Geometry check sheet. Reference: drawing and pictorial views, mm from the part's lowest x, y, z. A direction names the side the tool comes from. Coordinates: 2 decimals unless noted, no trailing zeros. Loops run counter-clockwise (first coordinate to the right, second up) from the corner with the lowest first, then second, coordinate; pieces in that order, holes last. Notation, with made-up numbers: (-10.75, 74) -> (-5.75, 74) arc R24 ccw to (-5.75, 106) -> close; hole circle Ø5 at (-22.5, 72). An arc over 180 degrees is marked (long way). Use CSV: the item, a comma, the result in double quotes.
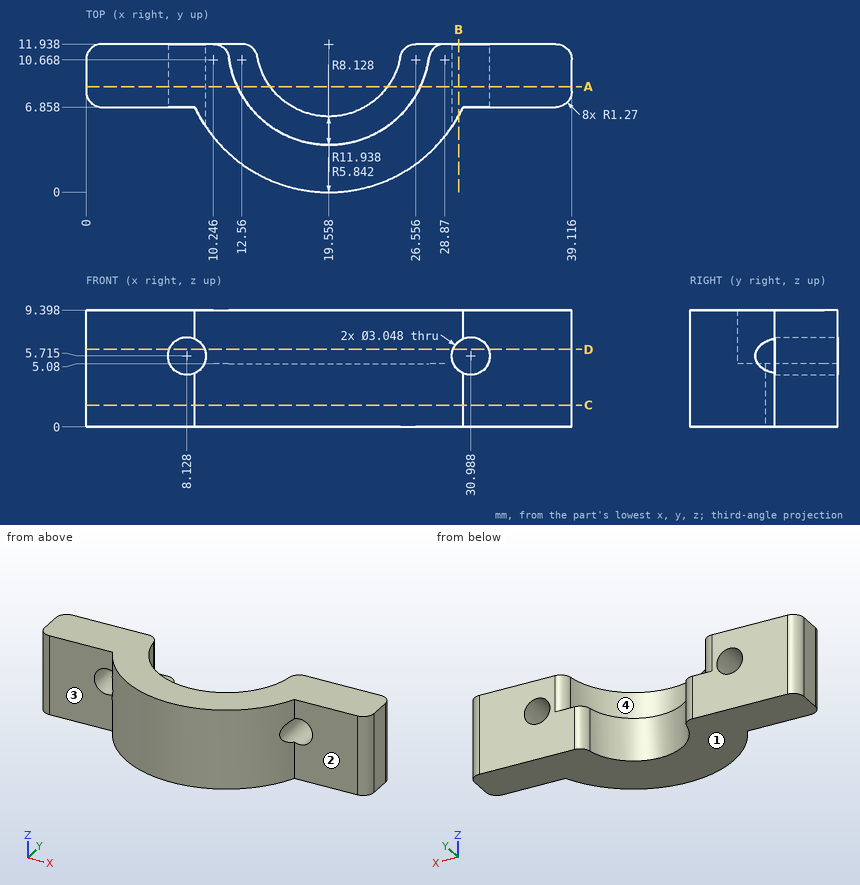
1) Thickness scan on line 1 along X through (y, z) = (9.5, 5.5) (1 decimal); line 2 along Y through (x, z) = (6.5, 6.5); line 3 along X through (y, z) = (8, 3.5) (1 decimal). Record the ranges inside material, lowest first. Write a range as from..to.
Answer below:
line 1,"x = 0..6.6, 9.6..11.8, 27.3..29.5, 32.5..39.1"
line 2,"y = 6.86..11.94"
line 3,"x = 0..15.2, 23.9..39.1"
2) Cross-section at D-D on z = 6.25. Record the boundary of the cut face in (x, y) (1 decimal).
Answer below:
outline,"(0, 8.1) arc R1.3 ccw to (1.3, 6.9) -> (6.7, 6.9) -> (6.7, 11.9) -> (1.3, 11.9) arc R1.3 ccw to (0, 10.7) -> close; (9.6, 5.4) arc R11.9 ccw to (29.6, 5.4) -> (29.6, 11.9) -> (28.9, 11.9) arc R1.3 ccw to (27.6, 10.8) arc R8.1 cw to (11.5, 10.8) arc R1.3 ccw to (10.2, 11.9) -> (9.6, 11.9) -> close; (32.4, 6.9) -> (37.8, 6.9) arc R1.3 ccw to (39.1, 8.1) -> (39.1, 10.7) arc R1.3 ccw to (37.8, 11.9) -> (32.4, 11.9) -> close"
3) Access from +Z, -Z, +X, -X, +Y, -Y to the whole of each face (thin tool, end or side, straight path). Record for the marked faces 1, 2, 3 and 4.
Answer below:
face 1,"-Z, +X, -X, +Y, -Y"
face 2,"+Z, -Z, +X, -Y"
face 3,"+Z, -Z, -X, -Y"
face 4,"+Z, +Y"
4) Cross-section at C-C on z = 1.75. Record the boundary of the cut face in (x, y) (1 decimal).
Answer below:
outline,"(0, 8.1) arc R1.3 ccw to (1.3, 6.9) -> (8.8, 6.9) arc R11.9 ccw to (30.4, 6.9) -> (37.8, 6.9) arc R1.3 ccw to (39.1, 8.1) -> (39.1, 10.7) arc R1.3 ccw to (37.8, 11.9) -> (26.6, 11.9) arc R1.3 ccw to (25.3, 10.9) arc R5.8 cw to (13.8, 10.9) arc R1.3 ccw to (12.6, 11.9) -> (1.3, 11.9) arc R1.3 ccw to (0, 10.7) -> close"
5) Cross-section at A-A on y = 8.5. Record the boundary of the cut face in (x, z) (1 decimal).
Answer below:
outline,"(0, 0) -> (14.8, 0) -> (14.8, 5.1) -> (12.2, 5.1) -> (12.2, 9.4) -> (0, 9.4) -> close; (24.3, 0) -> (39.1, 0) -> (39.1, 9.4) -> (26.9, 9.4) -> (26.9, 5.1) -> (24.3, 5.1) -> close; hole circle Ø3 at (8.1, 5.7); hole circle Ø3 at (31, 5.7)"
6) Go/stop test with flat-tipped pins: pin 1 Ø1.5 at (x, z) = (10, 4) entering from -Y; pin 2 Ø2.5 at (x, z) = (8.128, 5.715) entering from -Y; pin 3 Ø2 at (x, z) = (22, 3.5) entering from -Y. Record where each tip stops, or that it passes through.
Answer below:
pin 1,"stops at y = 3.88"
pin 2,"passes through"
pin 3,"stops at y = 0.09"
7) Cross-section at B-B on x = 30. Record the boundary of the cut face in (y, z) (1 decimal).
Answer below:
outline,"(6.2, 0) -> (11.9, 0) -> (11.9, 4.6) -> (6.2, 4.6) -> close; (6.2, 6.9) -> (11.9, 6.9) -> (11.9, 9.4) -> (6.2, 9.4) -> close"
